Can you work these out from the model? Positions are in its coordinate system, mm. Face numbers are marked on the shaded views. A direction names the side the tool comes from. Give positions to 0.01 mm unless a question says otherwise; leave off trailing zeros. Write each loop counter-clockwise with the first axis right and the second up, starting at its lowest first coordinate (ties: lowest second). Pieces come first, ordered by that corner, then holes. Notation, with made-up numbers: (57.5, 70) -> (110.5, 70) arc R24 ccw to (110.5, 94) -> close; hole circle Ø1 at (46.25, -25). An arc over 180 degrees is marked (long way). Answer as CSV lines item,"result". Start each with the question number.
1. If we section it at A-A on x = 0: Write out the boundary of the cut face in (y, z), plus the area to 3 significant figures.
2. If we mould it in two halves opening along Z, with no side actions, what happens to the marked faces 1, 2 and 3? For each: pulls with the +Z half, pulls with the -Z half, needs draft (parallel to the pull), parting line crosses it, or undercut.
3. On a 3-axis mill with a long thin cutter (end or side, diameter ignored), from which of +Z, -Z, +X, -X, +Y, -Y can I reach the whole of each face in a straight line? I mean the marked faces 4 and 5. Say none if no direction works.
4. I need wall thicknesses on line 1 (Y direction, x = 0, z = -2.25); line 2 (Y direction, x = 0, z = -2.7); line 3 (X direction, y = -9.75, z = -20.5). Which ranges of each line are inside material? Lowest first, please. Write a range as [from, to].
5. I'm going to push flat-ended pins straight in: P1, Ø8, axis at x = -16, z = -9.5, coming from the -Y side; P2, Ø6, axis at y = 6.5, z = -15.5, coming from the +X side; P3, Ø1.5, axis at x = -13.5, y = 5, coming from the -Z side. Where does each tip first touch, or does it pass through?
```python
from build123d import *

# Parameters (mm, degrees)
BOSS_EXTRUDE1_DEPTH     = 13.6525
CUT_EXTRUDE1_DEPTH      = 2.032
CUT_EXTRUDE9_DEPTH      = 0.127
FILLET3_R               = 2.54
FILLET4_R               = 2.54
SKETCH5_W               = 1.905
SKETCH5_H               = 23.241
CUT_EXTRUDE4_DEPTH      = 1.397
SKETCH6_W               = 1.905
SKETCH6_H               = 23.241
CUT_EXTRUDE5_DEPTH      = 1.397
SKETCH32_R              = 5.9944
BOSS_EXTRUDE4_DEPTH     = 1.5494
F_12_28_TAPPED_HOLE1_D  = 4.6228
SKETCH33_R              = 4.7625
SKETCH33_R_2            = 1.143
CUT_EXTRUDE16_DEPTH     = 1.0414
SKETCH34_R              = 8.7503
BOSS_EXTRUDE5_DEPTH     = 1.016
F_1_2_28_TAPPED_HOLE2_D = 11.811
CUT_EXTRUDE10_DEPTH     = 50.368791583
SKETCH27_R              = 3.7084
BOSS_EXTRUDE3_DEPTH     = 6.223
CUT_EXTRUDE13_DEPTH     = 1.143
SKETCH31_R              = 2.6416
CUT_EXTRUDE15_DEPTH     = 40.985274843
FILLET5_R               = 0.79375
FILLET6_R               = 1.905
FILLET7_R               = 0.381


with BuildPart() as part:
    # Sketch1 → Boss-Extrude1 (new, symmetric)
    with BuildSketch(Plane(origin=(0, 0, 0), x_dir=(1, 0, 0), z_dir=(0, 1, 0))):
        Polygon((-12.956855136, 0), (12.956855136, 0), (31.280615395, 18.323760259), (31.280615395, 22.768760259), (28.740615395, 22.768760259), (28.740615395, 19.375862707), (11.904752688, 2.54), (-12.508984605, 2.54), (-28.383984605, 8.318027469), (-28.383984605, 10.984500322), (-30.923984605, 10.984500322), (-30.923984605, 6.539500322), align=None)
    extrude(amount=BOSS_EXTRUDE1_DEPTH, both=True)

    # Sketch2 → Cut-Extrude1 (cut)
    with BuildSketch(Plane.XZ.offset(13.6525)):
        Polygon((12.378198789, -1.397), (29.883615395, -18.902416606), (29.883615395, -22.768760259), (31.280615395, -22.768760259), (31.280615395, -18.323760259), (12.956855136, 0), (-12.956855136, 0), (-30.923984605, -6.539500322), (-30.923984605, -10.984500322), (-29.526984605, -10.984500322), (-29.526984605, -7.517690253), (-12.710526344, -1.397), align=None)
    cut_extrude1 = extrude(amount=-CUT_EXTRUDE1_DEPTH, mode=Mode.SUBTRACT)

    # Sketch17 → Cut-Extrude9 (cut)
    with BuildSketch(Plane.XZ.offset(13.6525)):
        Polygon((28.740615395, -22.768760259), (29.883615395, -22.768760259), (29.883615395, -18.902416606), (12.378198789, -1.397), (-12.710526344, -1.397), (-29.526984605, -7.517690253), (-29.526984605, -10.984500322), (-28.383984605, -10.984500322), (-28.383984605, -8.318027469), (-12.508984605, -2.54), (11.904752688, -2.54), (28.740615395, -19.375862707), align=None)
    cut_extrude9 = extrude(amount=-CUT_EXTRUDE9_DEPTH, mode=Mode.SUBTRACT)

    # Mirror1: Cut-Extrude1, Cut-Extrude9 across plane
    add(cut_extrude1.mirror(Plane.ZX), mode=Mode.SUBTRACT)
    add(cut_extrude9.mirror(Plane.ZX), mode=Mode.SUBTRACT)

    # Fillet3
    fillet3_edges = [part.edges().sort_by_distance(p)[0] for p in [
        (-30.923984605, 0, -6.539500322),
        (31.280615395, 0, -18.323760259),
        (12.956855136, 0, 0),
        (-12.956855136, 0, 0),
        (-29.526984605, 12.573, -7.517690253),
        (-12.710526344, 12.573, -1.397),
        (12.378198789, 12.573, -1.397),
        (29.883615395, 12.573, -18.902416606),
        (29.883615395, -12.573, -18.902416606),
        (12.378198789, -12.573, -1.397),
        (-12.710526344, -12.573, -1.397),
        (-29.526984605, -12.573, -7.517690253),
    ]]
    fillet(fillet3_edges, radius=FILLET3_R)

    # Fillet4
    fillet4_edges = [part.edges().sort_by_distance(p)[0] for p in [
        (-28.383984605, 0, -8.318027469),
        (-12.508984605, 0, -2.54),
        (11.904752688, 0, -2.54),
        (28.740615395, 0, -19.375862707),
    ]]
    fillet(fillet4_edges, radius=FILLET4_R)

    # Sketch5 → Cut-Extrude4 (cut)
    with BuildSketch(Plane(origin=(31.280615395, 0, 0), x_dir=(0, 0, -1), z_dir=(1, 0, 0))):
        with Locations((21.816260259, 0)):
            Rectangle(SKETCH5_W, SKETCH5_H)
    extrude(amount=-CUT_EXTRUDE4_DEPTH, mode=Mode.SUBTRACT)

    # Sketch6 → Cut-Extrude5 (cut)
    with BuildSketch(Plane.ZY.offset(30.923984605)):
        with Locations((-10.032000322, 0)):
            Rectangle(SKETCH6_W, SKETCH6_H)
    extrude(amount=-CUT_EXTRUDE5_DEPTH, mode=Mode.SUBTRACT)

    # Sketch32 → Boss-Extrude4 (add)
    with BuildSketch(Plane(origin=(-0.646932965, 0, 1.777433714), x_dir=(-0.9396926207859079, 0, -0.3420201433256701), z_dir=(0.3420201433256701, 0, -0.9396926207859079))):
        with Locations(Location((20.404914452, -3.81, 0), (0, 0, 180))):
            Circle(SKETCH32_R)
    extrude(amount=BOSS_EXTRUDE4_DEPTH)

    # #12-28 Tapped Hole1 (through all)
    with Locations(Plane(origin=(-0.117006955, 0, 0.321473968), x_dir=(0.9396926207859079, 0, 0.3420201433256701), z_dir=(0.3420201433256701, 0, -0.9396926207859079))):
        with Locations((-20.404914452, 3.81)):
            Hole(F_12_28_TAPPED_HOLE1_D / 2)

    # Sketch33 → Cut-Extrude16 (cut)
    with BuildSketch(Plane(origin=(-1.515664129, 0, 4.164252971), x_dir=(0.9396926207859079, 0, 0.34202014332567005), z_dir=(-0.34202014332567005, 0, 0.9396926207859079))):
        with Locations((-20.404914452, -3.81)):
            Circle(SKETCH33_R)
        with Locations((-20.404914452, 2.8448)):
            Circle(SKETCH33_R_2)
    extrude(amount=-CUT_EXTRUDE16_DEPTH, mode=Mode.SUBTRACT)

    # Sketch34 → Boss-Extrude5 (add)
    with BuildSketch(Plane(origin=(0, 0, -2.54), x_dir=(-1, 0, 0), z_dir=(0, 0, -1))):
        with Locations(Location((0, -3.9751, 0), (0, 0, 180))):
            Circle(SKETCH34_R)
    extrude(amount=BOSS_EXTRUDE5_DEPTH)

    # 1/2-28 Tapped Hole2 (through all)
    with Locations(Plane(origin=(0, 0, -3.556), x_dir=(1, 0, 0), z_dir=(0, 0, -1))):
        with Locations((0, 3.9751)):
            Hole(F_1_2_28_TAPPED_HOLE2_D / 2)

    # Sketch22 → Cut-Extrude10 (cut, through all)
    with BuildSketch(Plane(origin=(6.478427568, 0, 6.478427568), x_dir=(0.7071067811865479, 0, -0.7071067811865472), z_dir=(0.7071067811865472, 0, 0.7071067811865479))):
        with BuildLine():
            Line((24.341545605, 6.6802), (19.895924926, 6.6802))
            ThreePointArc((19.895924926, 6.6802), (19.52095099, 6.677571434), (19.176049558, 6.53041382))
            ThreePointArc((19.176049558, 6.53041382), (14.955935265, 0), (19.176049558, -6.53041382))
            ThreePointArc((19.176049558, -6.53041382), (19.52095099, -6.677571434), (19.895924926, -6.6802))
            Line((19.895924926, -6.6802), (24.341545605, -6.6802))
            ThreePointArc((24.341545605, -6.6802), (24.716519541, -6.677571434), (25.061420973, -6.53041382))
            ThreePointArc((25.061420973, -6.53041382), (29.281535265, 0), (25.061420973, 6.53041382))
            ThreePointArc((25.061420973, 6.53041382), (24.716519541, 6.677571434), (24.341545605, 6.6802))
        make_face()
    extrude(amount=-CUT_EXTRUDE10_DEPTH, mode=Mode.SUBTRACT)

    # Sketch27 → Boss-Extrude3 (add)
    with BuildSketch(Plane(origin=(-0.646932965, 0, 1.777433714), x_dir=(-0.9396926207859079, 0, -0.3420201433256701), z_dir=(0.3420201433256701, 0, -0.9396926207859079))):
        with Locations(Location((17.414602222, 8.3439, 0), (0, 0, 180))):
            Circle(SKETCH27_R)
    extrude(amount=BOSS_EXTRUDE3_DEPTH)

    # Sketch30 → Cut-Extrude13 (cut)
    with BuildSketch(Plane(origin=(1.481458387, 0, -4.070273465), x_dir=(-0.9396926207859079, 0, -0.34202014332567005), z_dir=(0.34202014332567005, 0, -0.9396926207859079))):
        with BuildLine():
            Line((16.146138227, 10.9855), (18.683066217, 10.9855))
            ThreePointArc((18.683066217, 10.9855), (18.999757633, 10.976126048), (19.2627898, 10.799503844))
            ThreePointArc((19.2627898, 10.799503844), (17.414602222, 5.2705), (15.566414644, 10.799503844))
            ThreePointArc((15.566414644, 10.799503844), (15.829446811, 10.976126048), (16.146138227, 10.9855))
        make_face()
    extrude(amount=-CUT_EXTRUDE13_DEPTH, mode=Mode.SUBTRACT)

    # Sketch31 → Cut-Extrude15 (cut, through all)
    with BuildSketch(Plane(origin=(1.090529363, 0, -2.996204799), x_dir=(-0.9396926207859079, 0, -0.34202014332567005), z_dir=(0.34202014332567005, 0, -0.9396926207859079))):
        with Locations((17.414602222, 8.3439)):
            Circle(SKETCH31_R)
    extrude(amount=-CUT_EXTRUDE15_DEPTH, mode=Mode.SUBTRACT)

    # Fillet5
    fillet5_edges = [part.edges().sort_by_distance(p)[0] for p in [
        (-20.496062282, 8.3439, -5.447058533),
    ]]
    fillet(fillet5_edges, radius=FILLET5_R)

    # Fillet6
    # the kernel refuses this fillet: 1.905 mm, written as the material it takes off along each edge
    with BuildSketch(Plane(origin=(29.883615395, 17.890403349, -22.768760259), x_dir=(-1.0, 0, 7.382060356189012e-12), z_dir=(0, -1, 0)), Plane(origin=(-29.526984605, -17.890403349, -10.984500322), x_dir=(1.0, 0, 7.405372125734756e-12), z_dir=(0, 1, 0))) as fillet6_piece_1:
        with BuildLine():
            CenterArc((1.905, -1.74596134), FILLET6_R, 113.578178479, 66.421821522)
            Line((0, -1.74596134), (-0.0381, -1.74596134))
            Line((-0.0381, -1.74596134), (-0.0381, 0))
            Line((-0.0381, 0), (0, 0.0381))
            ThreePointArc((0, 0.0381), (0.5715, 0.0381), (1.12776, 0.034919227))
            Line((1.12776, 0.034919227), (1.143, 0))
        make_face()
    extrude(amount=35.780806699, mode=Mode.SUBTRACT)

    # Fillet7
    fillet7_edges = [part.edges().sort_by_distance(p)[0] for p in [
        (-28.383984605, 0, -10.984500322),
        (28.740615395, 0, -22.768760259),
    ]]
    fillet(fillet7_edges, radius=FILLET7_R)


solid = part.part
```
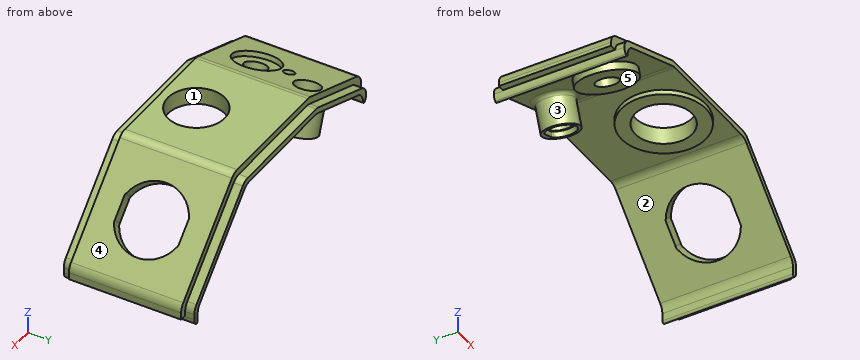
Computed values:
1,outline,"(-13.53, -2.54) -> (-12.73, -2.54) -> (-12.73, -3.56) -> (-9.88, -3.56) -> (-9.88, 0) -> (-11.62, 0) -> (-11.62, -1.4) -> (-13.53, -1.4) -> close; (1.93, -3.56) -> (4.78, -3.56) -> (4.78, -2.54) -> (13.53, -2.54) -> (13.53, -1.4) -> (11.62, -1.4) -> (11.62, 0) -> (1.93, 0) -> close"
1,area,"39.2 mm2"
2,face 1,"needs draft"
2,face 2,"pulls with the -Z half"
2,face 3,"undercut"
3,face 4,"+Z, +X, +Y, -Y"
3,face 5,"-Z, -Y"
4,line 1,"y = [-13.53, -9.88], [1.93, 13.53]"
4,line 2,"y = [-12.73, -9.88], [1.93, 4.78]"
4,line 3,"x = [28.74, 31.28]"
5,P1,"stops at y = -9.74"
5,P2,"stops at x = 31.12"
5,P3,"stops at z = -9.8"
